Part model, mm, in its own coordinate system. A direction names the side the tool comes from. Give positions to 0.01 mm unless a question says otherwise; leave off trailing zeros. Write each loop counter-clockwise with the first axis right and the second up, starting at its lowest first coordinate (ties: lowest second). Pieces come first, ordered by that corner, then holes.
Autodesk Inventor part; units mm, degrees
ref_plane "YZ Plane" through (0, 0, 0) normal (1, 0, 0) x (0, 1, 0)
ref_plane "XZ Plane" through (0, 0, 0) normal (0, 1, 0) x (-1, 0, 0)
ref_plane "XY Plane" through (0, 0, 0) normal (0, 0, 1) x (1, 0, 0)
sketch "スケッチ1" plane through (0, 0, 0) normal (0, 0, 1) x (1, 0, 0)
  circle A0 centre (0, 0) radius 7
  dimension "d0" = 14
extrude "押し出し1" add sketch "スケッチ1" along normal mid plane 48.5
sketch "スケッチ2" plane through (0, 0, 24.25) normal (0, 0, 1) x (1, 0, 0)
  circle A0 centre (0, 0) radius 2.65
  dimension "d3" = 5.3
extrude "押し出し2" add sketch "スケッチ2" along normal blind 1.7
fillet "フィレット1" radius 0.5 2 edges at (-7, 0, 24.25) (-7, 0, -24.25)
fillet "フィレット2" radius 0.2 2 edges at (-2.65, 0, 25.95) (-2.65, 0, 24.25)
properties part number "AA_Battery"
1) Wall check: L1, parallel to Z at x = 4.5, y = 2.25; L2, parallel to Y at x = 2.5, z = 10. Give the ranges that are in metal, low to high.
Answers follow:
L1: z = -24.25 to 24.25
L2: y = -6.54 to 6.54
2) 3-axis set-ups, long thin cutter, end or side, ignore diameter. For faces 1 (the face through (2.45, 1.01, 25.09)), 2 (the face through (6.466, -2.681, 0.332)): which of +Z, -Z, +X, -X, +Y, -Y reach the whole face in a straight line?
Answers follow:
face 1: +Z
face 2: +Z, -Z
3) Pin check, flat tips, straight feed: pin 1 Ø3 at (y, z) = (-4.5, -18) entering from +X; pin 2 Ø6 at (x, y) = (0, 5.5) entering from +Z; pin 3 Ø4 at (x, z) = (4, 0) entering from -Y. Stop position of each tip, or through.
Answers follow:
pin 1: stops at x = 6.32
pin 2: stops at z = 25.94
pin 3: stops at y = -6.71
4) Saw through at C-C, the plane z = -18. Write the cut outline in (x, y), then the cut area to 3 significant figures.
Answers follow:
outline: circle Ø14 at (0, 0)
area: 154 mm2
5) Saw through at A-A, the plane y = 0. Write the cut outline in (x, z).
Answers follow:
outline: (-7, -23.75) arc R0.5 ccw to (-6.5, -24.25) - (6.5, -24.25) arc R0.5 ccw to (7, -23.75) - (7, 23.75) arc R0.5 ccw to (6.5, 24.25) - (2.85, 24.25) arc R0.2 cw to (2.65, 24.45) - (2.65, 25.75) arc R0.2 ccw to (2.45, 25.95) - (-2.45, 25.95) arc R0.2 ccw to (-2.65, 25.75) - (-2.65, 24.45) arc R0.2 cw to (-2.85, 24.25) - (-6.5, 24.25) arc R0.5 ccw to (-7, 23.75) - close
